```python
from build123d import *

# Parameters (mm, degrees)
SKETCH1_R           = 6.5
SKETCH1_R_2         = 4
BOSS_EXTRUDE1_DEPTH = 12
BOSS_EXTRUDE2_START = -3
SKETCH2_R           = 1.15
BOSS_EXTRUDE2_DEPTH = 3
SKETCH4_R           = 6.5
SKETCH4_R_2         = 5
CUT_EXTRUDE1_DEPTH  = 2
BOSS_EXTRUDE4_START = -10
BOSS_EXTRUDE4_DEPTH = 10
CHAMFER1_SIZE       = 1.5


with BuildPart() as part:
    # Sketch1 → Boss-Extrude1 (new body)
    with BuildSketch(Plane(origin=(0, 0, 0), x_dir=(1, 0, 0), z_dir=(0, 1, 0))):
        with Locations(Location((0, 0, 0), (0, 0, 270))):
            Circle(SKETCH1_R)
        with Locations(Location((0, 0, 0), (0, 0, 270))):
            Circle(SKETCH1_R_2, mode=Mode.SUBTRACT)
    extrude(amount=BOSS_EXTRUDE1_DEPTH)

    # Sketch2 → Boss-Extrude2 (add)
    with BuildSketch(Plane(origin=(0, 12, 0), x_dir=(1, 0, 0), z_dir=(0, 1, 0)).offset(BOSS_EXTRUDE2_START)):
        with BuildLine():
            Line((22.477272727, 2.961791813), (1.034090909, 6.417215595))
            ThreePointArc((1.034090909, 6.417215595), (4.948312384, 4.214760319), (6.5, 0))
            ThreePointArc((6.5, 0), (4.948312384, -4.214760319), (1.034090909, -6.417215595))
            Line((1.034090909, -6.417215595), (22.477272727, -2.961791813))
            ThreePointArc((22.477272727, -2.961791813), (25, 0), (22.477272727, 2.961791813))
        make_face()
        with Locations(Location((22, 0, 0), (0, 0, 270))):
            Circle(SKETCH2_R, mode=Mode.SUBTRACT)
    extrude(amount=BOSS_EXTRUDE2_DEPTH)

    # Sketch4 → Cut-Extrude1 (cut)
    with BuildSketch(Plane.XZ):
        with Locations(Location((0, 0, 0), (0, 0, 270))):
            Circle(SKETCH4_R)
        with Locations(Location((0, 0, 0), (0, 0, 270))):
            Circle(SKETCH4_R_2, mode=Mode.SUBTRACT)
    extrude(amount=-CUT_EXTRUDE1_DEPTH, mode=Mode.SUBTRACT)

    # Sketch5 → Boss-Extrude4 (add)
    with BuildSketch(Plane(origin=(0, 12, 0), x_dir=(1, 0, 0), z_dir=(0, 1, 0)).offset(BOSS_EXTRUDE4_START)):
        with BuildLine():
            Line((-0.60381401, -3.954163457), (-3.726313009, 1.454163457))
            ThreePointArc((-3.726313009, 1.454163457), (-3.464101615, -2), (-0.60381401, -3.954163457))
        make_face()
    extrude(amount=BOSS_EXTRUDE4_DEPTH)

    # Chamfer1
    chamfer1_edges = [part.edges().sort_by_distance(p)[0] for p in [
        (0, 2, 5),
    ]]
    chamfer(chamfer1_edges, length=CHAMFER1_SIZE - 0.0001)  # a hair under: the kernel refuses the full size


solid = part.part
```
Input: part model. Units: mm. Frame: model coordinates. A direction names the side the tool comes from. Round coordinates to 2 decimals unless told otherwise and drop trailing zeros. Loops run counter-clockwise (first coordinate to the right, second up) from the corner with the lowest first, then second, coordinate; pieces in that order, holes last.
1) Set-up query: faces 1 (the cylindrical face through (25, 10, 0)), 2 (the flat face through (-3, 2, 2)). Return all of +Z, -Z, +X, -X, +Y, -Y with unobstructed straight access to the full face (end or side cutting, diameter ignored); none if empty.
Ans:
face 1: +X, +Y, -Y
face 2: -Y
2) Pull-direction query (X, two-part tool) for faces 3 (the flat face through (-2.14, 6.93, 1.29)), 4 (the flat face through (11.606, 10.479, 4.714)), 5 (the cylindrical face through (-6.345, 5.819, -1.409)); classes: released by +X, released by -X, zero draft, split by the parting line, or undercut.
Ans:
face 3: undercut
face 4: released by +X
face 5: split by the parting line
3) Section query C-C on z = 0. Count the separate pieces of the cut face and the enclosed holes in it, plus the area to 3 significant figures.
Ans:
separate pieces: 3
enclosed holes: 0
area: 116 mm2
4) Section query D-D on y = 6.25. Return the cut outline in (x, z).
Ans:
outline: circle Ø13 at (0, 0); hole (-3.73, -1.45) arc R4 ccw (long way) to (-0.6, 3.95) - close
5) Section query B-B on y = 9.5. Return the cut outline in (x, z).
Ans:
outline: (1.03, -6.42) - (22.48, -2.96) arc R3 ccw to (22.48, 2.96) - (1.03, 6.42) arc R6.5 ccw (long way) to start; hole (-3.73, -1.45) arc R4 ccw (long way) to (-0.6, 3.95) - close; hole circle Ø2.3 at (22, 0)
6) Pin query (flat end, axial travel): pin 1 (4 mm diameter, centred on y = 10.5, z = 1.5, fed in from +X); pin 2 (4 mm diameter, centred on x = 10.5, z = 1, fed in from -Y); pin 3 (1.5 mm diameter, centred on y = 9, z = -5, fed in from -X); pin 4 (1.5 mm diameter, centred on y = 3.5, z = 2.5, fed in from +X). Return the tip coordinate at first contact, or that it passes through.
Ans:
pin 1: stops at x = 25
pin 2: stops at y = 9
pin 3: stops at x = -4.92
pin 4: stops at x = 6.26
7) Material intervals for line 1 (Y direction, x = 10, z = 1); line 2 (X direction, y = 10.3, z = 0); line 3 (Z direction, x = 1, y = 1.75), sorted ascending.
Ans:
line 1: y = 9 to 12
line 2: x = -6.5 to -2.89, 4 to 20.85, 23.15 to 25
line 3: z = -6.17 to -3.87, 3.87 to 6.17
